Work out the finished part from the listing and answer in its coordinate system (mm). A direction names the side the tool comes from. Give positions to 0.01 mm unless a question says otherwise; leave off trailing zeros. Order: outer loops, then holes, each group sorted by start corner. A loop starts at its lowest first (then second) coordinate and runs counter-clockwise, first axis right, second up. Notation, with made-up numbers: (57.5, 6.5) - (71.5, 6.5) arc R7 cw to (71.5, 18.5) - close; hole circle Ø2 at (21.25, 22.25). An arc over 180 degrees is marked (long way). Write each question's results on one line, items separated by ' | '.
from build123d import *

# Parameters (mm, degrees)
SKETCH2_W            = 46
SKETCH2_H            = 38
SKETCH2_R            = 1.5
BOSS_EXTRUDE1_DEPTH  = 1.5
SKETCH12_W           = 21
SKETCH12_H           = 20
BOSS_EXTRUDE6_DEPTH  = 12
SKETCH13_W           = 18
SKETCH13_H           = 12
BOSS_EXTRUDE7_DEPTH  = 2
SKETCH15_W           = 30
SKETCH15_H           = 12
BOSS_EXTRUDE8_DEPTH  = 6.5
SKETCH16_W           = 10
SKETCH16_H           = 11.5
BOSS_EXTRUDE9_DEPTH  = 23
SKETCH17_W           = 8
SKETCH17_H           = 11.5
BOSS_EXTRUDE10_DEPTH = 23
SKETCH18_W           = 12
SKETCH18_H           = 8.151595729
BOSS_EXTRUDE11_DEPTH = 18
SKETCH19_W           = 9.5
SKETCH19_H           = 11
CUT_EXTRUDE3_DEPTH   = 16.5
SKETCH22_W           = 7
SKETCH22_H           = 10.75
CUT_EXTRUDE4_DEPTH   = 16.5


with BuildPart() as part:
    # Sketch2 → Boss-Extrude1 (new body)
    with BuildSketch(Plane.XY):
        with Locations((23, 19)):
            Rectangle(SKETCH2_W, SKETCH2_H)
        with Locations((4.5, 28)):
            Circle(SKETCH2_R, mode=Mode.SUBTRACT)
        with Locations((4.5, 5.5)):
            Circle(SKETCH2_R, mode=Mode.SUBTRACT)
        with Locations((41.5, 5.5)):
            Circle(SKETCH2_R, mode=Mode.SUBTRACT)
        with Locations((41.5, 28)):
            Circle(SKETCH2_R, mode=Mode.SUBTRACT)
    extrude(amount=BOSS_EXTRUDE1_DEPTH)

    # Sketch12 → Boss-Extrude6 (add)
    with BuildSketch(Plane.XY):
        with Locations((23, 28)):
            Rectangle(SKETCH12_W, SKETCH12_H)
    extrude(amount=-BOSS_EXTRUDE6_DEPTH)

    # Sketch13 → Boss-Extrude7 (add)
    with BuildSketch(Plane.XY):
        with Locations((23, 27.789125994)):
            Rectangle(SKETCH13_W, SKETCH13_H)
    extrude(amount=BOSS_EXTRUDE7_DEPTH)

    # Sketch15 → Boss-Extrude8 (add)
    with BuildSketch(Plane.XY):
        with Locations((23, 6)):
            Rectangle(SKETCH15_W, SKETCH15_H)
    extrude(amount=BOSS_EXTRUDE8_DEPTH)

    # Sketch16 → Boss-Extrude9 (add)
    with BuildSketch(Plane.XY):
        with Locations((13, 6)):
            Rectangle(SKETCH16_W, SKETCH16_H)
    extrude(amount=BOSS_EXTRUDE9_DEPTH)

    # Sketch17 → Boss-Extrude10 (add)
    with BuildSketch(Plane.XY):
        with Locations((34, 6)):
            Rectangle(SKETCH17_W, SKETCH17_H)
    extrude(amount=BOSS_EXTRUDE10_DEPTH)

    # Sketch18 → Boss-Extrude11 (add)
    with BuildSketch(Plane.XY):
        with Locations((24, 6.075797865)):
            Rectangle(SKETCH18_W, SKETCH18_H)
    extrude(amount=BOSS_EXTRUDE11_DEPTH)

    # Sketch19 → Cut-Extrude3 (cut)
    with BuildSketch(Plane.XY.offset(17)):
        with Locations((13, 6)):
            Rectangle(SKETCH19_W, SKETCH19_H)
    extrude(amount=CUT_EXTRUDE3_DEPTH, mode=Mode.SUBTRACT)

    # Sketch22 → Cut-Extrude4 (cut)
    with BuildSketch(Plane.XY.offset(12)):
        with Locations((34, 5.875)):
            Rectangle(SKETCH22_W, SKETCH22_H)
    extrude(amount=CUT_EXTRUDE4_DEPTH, mode=Mode.SUBTRACT)


solid = part.part
1. Determine the mould class of faces 1 (the face through (34, 0.25, 15)), 2 (the face through (34, 11.25, 17)), 3 (the face through (38, 6, 12)) for opening direction X: +X half, -X half, draft (parallel to the pull), parting line (faces both ways), or undercut.
Answer list:
face 1: draft | face 2: undercut | face 3: +X half
2. Given P1, Ø2.5, axis at x = 41.5, y = 28, coming from the -Z side; P2, Ø1, axis at y = 10, z = 8.5, coming from the -X side; P3, Ø5, axis at x = 4.5, y = 5.5, coming from the +Z side; P4, Ø8.5, axis at y = 7.5, z = 18.5, coming from the +X side, each flat-ended and moving along its own axis, determine where each tip first touches the part or whether it passes through.
Answer list:
P1: through | P2: x = 8 | P3: z = 1.5 | P4: x = 38
3. A cutting plane is placed at B-B, the plane z = 14. Write down the section's boundary in (x, y).
Answer list:
outline: (8, 0.25) - (18, 0.25) - (18, 2) - (30, 2) - (30, 0.25) - (38, 0.25) - (38, 11.75) - (30, 11.75) - (30, 10.15) - (18, 10.15) - (18, 11.75) - (8, 11.75) - close; hole (30.5, 0.5) - (37.5, 0.5) - (37.5, 11.25) - (30.5, 11.25) - close
4. A tool of negligible diameter and unlimited length cuts with its end or side. For faces 4 (the face through (33.5, 28, -6)), 5 (the face through (8, 6, 12)), 6 (the face through (34, 6, 12)), from which of +Z, -Z, +X, -X, +Y, -Y can it reach the whole face along a straight path? Write none if from no direction.
Answer list:
face 4: -Z, +X, +Y, -Y | face 5: +Z, -X, +Y, -Y | face 6: +Z
5. A cutting plane is placed at D-D, the plane x = 36.5. Write down the section's boundary in (y, z).
Answer list:
outline: (0, 0) - (38, 0) - (38, 1.5) - (12, 1.5) - (12, 6.5) - (11.75, 6.5) - (11.75, 23) - (11.25, 23) - (11.25, 12) - (0.5, 12) - (0.5, 23) - (0.25, 23) - (0.25, 6.5) - (0, 6.5) - close
6. Straight lines are drawn through the part: line 1 (Y direction, x = 4.5, z = 0.75); line 2 (X direction, y = 24, z = -9); line 3 (Z direction, x = 43, y = 18.5). For each, find the intervals that lie inside material, in ascending order. Write a range as [from, to].
Answer list:
line 1: [0, 4], [7, 26.5], [29.5, 38] | line 2: [12.5, 33.5] | line 3: [0, 1.5]
7. A cutting plane is placed at C-C, the plane x = 4.5. Write down the section's boundary in (y, z).
Answer list:
outline: (0, 0) - (4, 0) - (4, 1.5) - (0, 1.5) - close; (7, 0) - (26.5, 0) - (26.5, 1.5) - (7, 1.5) - close; (29.5, 0) - (38, 0) - (38, 1.5) - (29.5, 1.5) - close
8. A cutting plane is placed at A-A, the plane y = 5.5. Write down the section's boundary in (x, z), then the cut area to 3 significant figures.
Answer list:
outline: (0, 0) - (3, 0) - (3, 1.5) - (0, 1.5) - close; (6, 0) - (40, 0) - (40, 1.5) - (38, 1.5) - (38, 23) - (37.5, 23) - (37.5, 12) - (30.5, 12) - (30.5, 23) - (30, 23) - (30, 18) - (18, 18) - (18, 23) - (17.75, 23) - (17.75, 17) - (8.25, 17) - (8.25, 23) - (8, 23) - (8, 1.5) - (6, 1.5) - close; (43, 0) - (46, 0) - (46, 1.5) - (43, 1.5) - close | area: 511 mm^2
